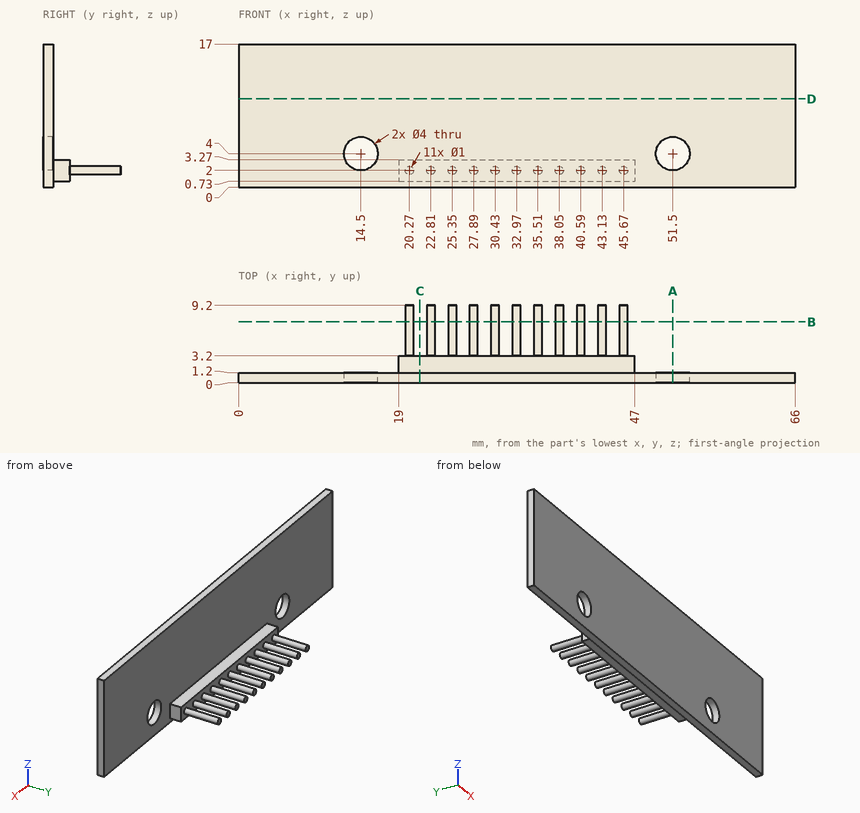
Answer from the drawing. Dimensions are ordinates in mm from the lowest x, y and z of the part. Give positions to 0.01 mm unless a question says otherwise; leave off trailing zeros. Loops run counter-clockwise (first coordinate to the right, second up) from the corner with the lowest first, then second, coordinate; pieces in that order, holes last. Notation, with made-up numbers: (-15, 26.25) - (23, 26.25) arc R18 cw to (23, 60.25) - close; hole circle Ø4 at (-21.5, 37.25). An arc over 180 degrees is marked (long way). Answer as CSV lines item,"result". Start each with the question number.
Item 1: A cutting plane is placed at B-B on y = 7.25. Count the separate pieces of the cut face and the enclosed holes in it, then the cut area to 3 significant figures.
Item 2: Find the intervals of material crossed by line 1 (X direction, y = 0.95, z = 4); line 2 (Z direction, x = 51.5, y = 0.65); line 3 (Y direction, x = 29.5, z = 4.75), in increasing order. Write a range as from..to.
Item 3: A cutting plane is placed at A-A on x = 51.5. Determine the outline of the cut face in (y, z), then the cut area to 3 significant figures.
Item 4: A cutting plane is placed at D-D on z = 10.5. Determine the outline of the cut face in (x, y), then the cut area to 3 significant figures.
Item 5: Each of these flat-tipped pins is pushed along its axis until it touches: pin 1 (4 mm diameter, centred on x = 48, z = 15, fed in from -Y); pin 2 (0.6 mm diameter, centred on y = 2, z = 2.5, fed in from +X); pin 3 (2 mm diameter, centred on x = 43.5, z = 13.5, fed in from +Y); pin 4 (1.5 mm diameter, centred on y = 3.5, z = 5, fed in from -X). Where does it stop, or does it pass through?
Item 6: A cutting plane is placed at C-C on x = 21.5. Determine the outline of the cut face in (y, z).
Found:
1,separate pieces,"11"
1,enclosed holes,"0"
1,area,"8.64 mm^2"
2,line 1,"x = 0..12.5, 16.5..49.5, 53.5..66"
2,line 2,"z = 0..2, 6..17"
2,line 3,"y = 0..1.2"
3,outline,"(0, 0) - (1.2, 0) - (1.2, 2) - (0, 2) - close; (0, 6) - (1.2, 6) - (1.2, 17) - (0, 17) - close"
3,area,"15.6 mm^2"
4,outline,"(0, 0) - (66, 0) - (66, 1.2) - (0, 1.2) - close"
4,area,"79.2 mm^2"
5,pin 1,"stops at y = 0"
5,pin 2,"stops at x = 47"
5,pin 3,"stops at y = 1.2"
5,pin 4,"passes through"
6,outline,"(0, 0) - (1.2, 0) - (1.2, 0.73) - (3.2, 0.73) - (3.2, 3.27) - (1.2, 3.27) - (1.2, 17) - (0, 17) - close"
